```python
from build123d import *

# Parameters (mm, degrees)
SKETCH1_W           = 25
SKETCH1_H           = 10
SKETCH2_R           = 20
BOSS_EXTRUDE1_DEPTH = 5
BOSS_EXTRUDE2_START = 5
SKETCH3_R           = 20
BOSS_EXTRUDE2_DEPTH = 5


with BuildPart() as part:
    # Sketch1 → Revolve1 (revolve)
    with BuildSketch(Plane.XY, mode=Mode.PRIVATE) as revolve1_sk:
        with Locations((0, 5)):
            Rectangle(SKETCH1_W, SKETCH1_H)
    revolve(revolve1_sk.sketch.rotate(Axis((0, 0, 0), (1, 0, 0)), 90), axis=Axis((0, 0, 0), (1, 0, 0)))

    # Sketch2 → Boss-Extrude1 (add)
    with BuildSketch(Plane.ZY.offset(12.5)):
        Circle(SKETCH2_R)
    extrude(amount=BOSS_EXTRUDE1_DEPTH)

    # Sketch3 → Boss-Extrude2 (add)
    with BuildSketch(Plane(origin=(12.5, 0, 0), x_dir=(0, 0, -1), z_dir=(1, 0, 0)).offset(BOSS_EXTRUDE2_START)):
        with Locations(Location((0, 0, 0), (0, 0, 180))):
            Circle(SKETCH3_R)
    extrude(amount=-BOSS_EXTRUDE2_DEPTH)


solid = part.part
```
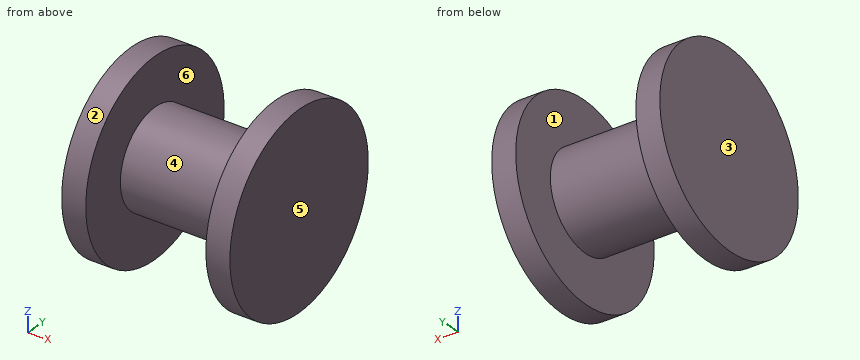
For this review, take the finished solid that the model builds, in its own axes (mm). Face numbers are marked on the shaded views. A direction names the side the tool comes from. Round coordinates to 2 decimals unless told otherwise and drop trailing zeros. Loops run counter-clockwise (first coordinate to the right, second up) from the corner with the lowest first, then second, coordinate; pieces in that order, holes last.
Q1. Add section C-C on x = -4. Write out the cut boundary in (y, z).
Result sheet:
outline: circle Ø20 at (0, 0)
Q2. Add section D-D on x = 14. Write out the cut boundary in (y, z), plus the area to 3 significant figures.
Result sheet:
outline: circle Ø40 at (0, 0)
area: 1,260 mm2
Q3. Add section A-A on z = 0. Write out the cut boundary in (x, y).
Result sheet:
outline: (-17.5, -20) - (-12.5, -20) - (-12.5, -10) - (12.5, -10) - (12.5, -20) - (17.5, -20) - (17.5, 20) - (12.5, 20) - (12.5, 10) - (-12.5, 10) - (-12.5, 20) - (-17.5, 20) - close
Q4. Machinability: for the marked faces 5 and 6, which of the approach directions +Z, -Z, +X, -X, +Y, -Y give a long, thin tool a straight path to every point of the face, cutting with its end or side? Answer none if there is none.
Result sheet:
face 5: +Z, -Z, +X, +Y, -Y
face 6: none
Q5. Mouldability with a two-part tool opening along X and no side actions: class the marked faces 1, 2, 3 and 4 as +X half, -X half, draft (parallel to the pull), parting line (faces both ways), or undercut.
Result sheet:
face 1: undercut
face 2: draft
face 3: -X half
face 4: undercut
Q6. Insertion check: pin 1 Ø4 at (x, y) = (14, -15) entering from +Z; pin 2 Ø5 at (x, z) = (-0.5, 4.5) entering from -Y; pin 3 Ø3 at (x, y) = (5, -1) entering from -Z. Each pin has a flat end and moves straight along its axis. Give the tip position at first contact, or say it passes through.
Result sheet:
pin 1: stops at z = 15.2
pin 2: stops at y = -9.8
pin 3: stops at z = -10
Q7. To check wall thickness, follow line 1 along X through (y, z) = (10.5, 11.5); line 2 along Y through (x, z) = (6, -4.5); line 3 along Z through (x, y) = (-14, 4). State the ranges of each line that lie inside material, in increasing order.
Result sheet:
line 1: x = -17.5 to -12.5, 12.5 to 17.5
line 2: y = -8.93 to 8.93
line 3: z = -19.6 to 19.6
Q8. Add section B-B on y = 5.5. Write out the cut boundary in (x, z), plus the area to 3 significant figures.
Result sheet:
outline: (-17.5, -19.23) - (-12.5, -19.23) - (-12.5, -8.35) - (12.5, -8.35) - (12.5, -19.23) - (17.5, -19.23) - (17.5, 19.23) - (12.5, 19.23) - (12.5, 8.35) - (-12.5, 8.35) - (-12.5, 19.23) - (-17.5, 19.23) - close
area: 802 mm2
